The model under review builds one solid part; all positions refer to its coordinate system, in mm. Face numbers are marked on the shaded views. A direction names the side the tool comes from. Coordinates: 2 decimals unless noted, no trailing zeros. Order: outer loops, then holes, each group sorted by start corner. A loop starts at its lowest first (then second) coordinate and runs counter-clockwise, first axis right, second up. Notation, with made-up numbers: M 69.25,-36.75 L 75.25,-36.75 A20 cw 75.25,-24.75 Z; hole C 7.5,5.25 d8. An arc over 180 degrees is marked long. Answer in a Markdown table with one row per item.
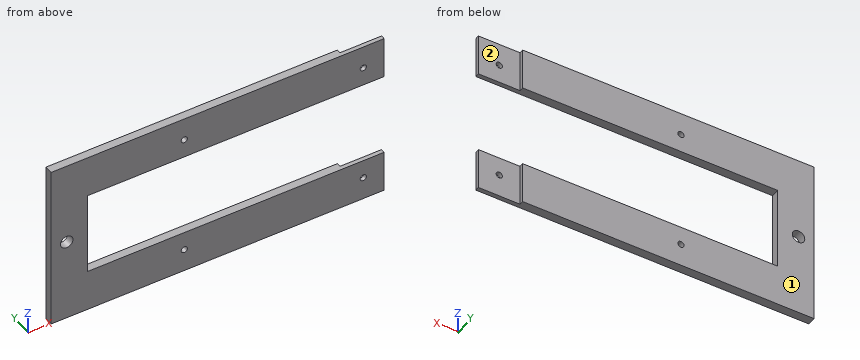
from build123d import *

# Parameters (mm, degrees)
SKETCH1_R           = 1.5
BOSS_EXTRUDE1_DEPTH = 4
SKETCH2_W           = 20
SKETCH2_H           = 2
CUT_EXTRUDE1_DEPTH  = 20


with BuildPart() as part:
    # Sketch1 → Boss-Extrude1 (new body)
    # profile 1 of 2: a face of its own
    with BuildSketch(Plane(origin=(0, 0, 0), x_dir=(1, 0, 0), z_dir=(0, 1, 0))):
        with BuildLine():
            Line((0, 0), (0, -40))
            Line((0, -40), (160, -40))
            Line((160, -40), (160, -20))
            Line((160, -20), (17.5, -20))
            Line((17.5, -20), (17.5, 0))
            Line((17.5, 0), (10.5, 0))
            ThreePointArc((10.5, 0), (7.5, -3), (4.5, 0))
            Line((4.5, 0), (0, 0))
        make_face()
        with Locations(Location((64, -29, 0), (0, 0, 270))):
            Circle(SKETCH1_R, mode=Mode.SUBTRACT)
        with Locations(Location((150, -29, 0), (0, 0, 270))):
            Circle(SKETCH1_R, mode=Mode.SUBTRACT)
    # profile 2 of 2: a face of its own
    with BuildSketch(Plane(origin=(0, 0, 0), x_dir=(1, 0, 0), z_dir=(0, 1, 0))):
        with BuildLine():
            Line((0, 40), (0, 0))
            Line((0, 0), (4.5, 0))
            ThreePointArc((4.5, 0), (7.5, 3), (10.5, 0))
            Line((10.5, 0), (17.5, 0))
            Line((17.5, 0), (17.5, 20))
            Line((17.5, 20), (160, 20))
            Line((160, 20), (160, 40))
            Line((160, 40), (0, 40))
        make_face()
        with Locations(Location((64, 29, 0), (0, 0, 270))):
            Circle(SKETCH1_R, mode=Mode.SUBTRACT)
        with Locations(Location((150, 29, 0), (0, 0, 270))):
            Circle(SKETCH1_R, mode=Mode.SUBTRACT)
    extrude(amount=BOSS_EXTRUDE1_DEPTH)

    # Sketch2 → Cut-Extrude1 (cut)
    with BuildSketch(Plane(origin=(160, 0, 0), x_dir=(0, 0, -1), z_dir=(1, 0, 0))):
        with Locations((30, 3)):
            Rectangle(SKETCH2_W, SKETCH2_H)
        with Locations((-30, 3)):
            Rectangle(SKETCH2_W, SKETCH2_H)
    extrude(amount=-CUT_EXTRUDE1_DEPTH, mode=Mode.SUBTRACT)


solid = part.part
(1) Take a section at B-B (x = 64). Write out the cut boundary in (y, z).
Report:
| item | result |
|---|---|
| outline | M 0,-40 L 4,-40 L 4,-30.5 L 0,-30.5 Z; M 0,-27.5 L 4,-27.5 L 4,-20 L 0,-20 Z; M 0,20 L 4,20 L 4,27.5 L 0,27.5 Z; M 0,30.5 L 4,30.5 L 4,40 L 0,40 Z |
(2) Machinability: for the marked faces 1 and 2, which of the approach directions +Z, -Z, +X, -X, +Y, -Y give a long, thin tool a straight path to every point of the face, cutting with its end or side? Answer none if there is none.
Report:
| item | result |
|---|---|
| face 1 | +Z, -Z, +X, -X, +Y |
| face 2 | +Z, -Z, +X, +Y |
(3) Insertion check: P1, Ø1.5, axis at y = 2, z = 0, coming from the +X side; P2, Ø10, axis at x = 150.5, z = 32.5, coming from the +Y side; P3, Ø2, axis at y = 3.5, z = 33.5, coming from the +X side. Each pin has a flat end and moves straight along its axis. Give the tip position at first contact, or say it passes through.
Report:
| item | result |
|---|---|
| P1 | x = 17.5 |
| P2 | y = 2 |
| P3 | x = 140 |
(4) Take a section at D-D (x = 7.5). Write out the cut boundary in (y, z).
Report:
| item | result |
|---|---|
| outline | M 0,-40 L 4,-40 L 4,-3 L 0,-3 Z; M 0,3 L 4,3 L 4,40 L 0,40 Z |
(5) To check wall thickness, follow line 1 (Z direction, x = 64, y = 2.6); line 2 (X direction, y = 0.5, z = -29); line 3 (Z direction, x = 128, y = 3.4). State the ranges of each line that lie inside material, in increasing order. Write a range as [from, to].
Report:
| item | result |
|---|---|
| line 1 | [-40, -30.5], [-27.5, -20], [20, 27.5], [30.5, 40] |
| line 2 | [0, 62.5], [65.5, 148.5], [151.5, 160] |
| line 3 | [-40, -20], [20, 40] |
(6) Take a section at A-A (z = -29). Write out the cut boundary in (x, y), then the cut area to 3 significant figures.
Report:
| item | result |
|---|---|
| outline | M 0,0 L 62.5,0 L 62.5,4 L 0,4 Z; M 65.5,0 L 148.5,0 L 148.5,2 L 140,2 L 140,4 L 65.5,4 Z; M 151.5,0 L 160,0 L 160,2 L 151.5,2 Z |
| area | 582 mm^2 |
(7) Take a section at C-C (y = 1.3). Write out the cut boundary in (x, z), then the cut area to 3 significant figures.
Report:
| item | result |
|---|---|
| outline | M 0,-40 L 160,-40 L 160,-20 L 17.5,-20 L 17.5,20 L 160,20 L 160,40 L 0,40 Z; hole C 7.5,0 d6; hole C 64,-29 d3; hole C 64,29 d3; hole C 150,-29 d3; hole C 150,29 d3 |
| area | 7,040 mm^2 |
